For this review, take the finished solid that the model builds, in its own axes (mm). A direction names the side the tool comes from. Round coordinates to 2 decimals unless told otherwise and drop trailing zeros. Write each loop counter-clockwise with the first axis right and the second up, starting at its lowest first coordinate (ties: lowest second). Pieces come first, ordered by that corner, then holes. Notation, with made-up numbers: (28.5, 70.25) -> (74.5, 70.25) arc R4 ccw to (74.5, 76.25) -> close; hole circle Ø5 at (-18, 45.5). An arc over 180 degrees is marked (long way). Answer in a Markdown table with one row per item.
from build123d import *

# Parameters (mm, degrees)
CUT_EXTRUDE1_REACH      = 219.495
CUT_EXTRUDE1_END_RADIUS = 7.5
SKETCH2_W               = 8
SKETCH2_H               = 13
CUT_EXTRUDE2_REACH      = 219.495
CUT_EXTRUDE2_END_RADIUS = 7.5
SKETCH2_3_W             = 4.6
SKETCH2_3_H             = 13


with BuildPart() as part:
    # Sketch1 → Revolve1 (revolve)
    with BuildSketch(Plane.XY, mode=Mode.PRIVATE) as revolve1_sk:
        Polygon((157, 6.5), (157, 7.5), (55, 7.5), (55, 18), (-55, 18), (-55, 7.5), (-216, 7.5), (-216, 6.5), align=None)
    revolve(revolve1_sk.sketch.rotate(Axis((196.356223274, 0, 0), (-1, 0, 0)), 90), axis=Axis((196.356223274, 0, 0), (-1, 0, 0)))

    # Cut-Extrude1: up to this cylinder (the profile starts inside it)
    cut_extrude1_end = Plane(origin=(-64, 0, 0), z_dir=(1, 0, 0)) * Cylinder(CUT_EXTRUDE1_END_RADIUS, 454.99, mode=Mode.PRIVATE)
    # Sketch2 → Cut-Extrude1 (cut, up to the surface)
    with BuildSketch(Plane(origin=(0, 0, 0), x_dir=(1, 0, 0), z_dir=(0, 1, 0)), mode=Mode.PRIVATE) as cut_extrude1_sk1:
        with Locations((-64, 0)):
            Rectangle(SKETCH2_W, SKETCH2_H)
    cut_extrude1_tool1 = extrude(cut_extrude1_sk1.sketch, amount=-CUT_EXTRUDE1_REACH, mode=Mode.PRIVATE) & cut_extrude1_end
    add(cut_extrude1_tool1.solids().sort_by_distance((-64, 0, 0))[0], mode=Mode.SUBTRACT)

    # Cut-Extrude2: up to this cylinder (the profile starts inside it)
    cut_extrude2_end = Plane(origin=(-183.3, 0, 0), z_dir=(1, 0, 0)) * Cylinder(CUT_EXTRUDE2_END_RADIUS, 454.99, mode=Mode.PRIVATE)
    # Sketch2<3> → Cut-Extrude2 (cut, up to the surface)
    with BuildSketch(Plane(origin=(0, 0, 0), x_dir=(1, 0, 0), z_dir=(0, 1, 0)), mode=Mode.PRIVATE) as cut_extrude2_sk1:
        with Locations((-183.3, 0)):
            Rectangle(SKETCH2_3_W, SKETCH2_3_H)
    cut_extrude2_tool1 = extrude(cut_extrude2_sk1.sketch, amount=CUT_EXTRUDE2_REACH, mode=Mode.PRIVATE) & cut_extrude2_end
    add(cut_extrude2_tool1.solids().sort_by_distance((-183.3, 0, 0))[0], mode=Mode.SUBTRACT)


solid = part.part
1) Consider section A-A on z = 0. State the section outline as (x, y) points, then the cut area to 3 significant figures.
Solved:
| item | result |
|---|---|
| outline | (-216, -7.5) -> (-68, -7.5) -> (-68, -6.5) -> (-216, -6.5) -> close; (-216, 6.5) -> (-185.6, 6.5) -> (-185.6, 7.5) -> (-216, 7.5) -> close; (-181, 6.5) -> (157, 6.5) -> (157, 7.5) -> (55, 7.5) -> (55, 18) -> (-55, 18) -> (-55, 7.5) -> (-181, 7.5) -> close; (-60, -7.5) -> (-55, -7.5) -> (-55, -18) -> (55, -18) -> (55, -7.5) -> (157, -7.5) -> (157, -6.5) -> (-60, -6.5) -> close |
| area | 3,040 mm² |
2) Clearance check with flat-ended pins moving along their axes: pin 1 Ø6 at (x, z) = (34.5, -10) entering from -Y; pin 2 Ø4 at (x, y) = (-63, -2.5) entering from -Z; pin 3 Ø3 at (x, y) = (0, -12) entering from +Z; pin 4 Ø4 at (y, z) = (-2, -1.5) entering from -X. State where each tip first meets the part, or that it passes through.
Solved:
| item | result |
|---|---|
| pin 1 | y = -16.58 |
| pin 2 | z = -7.48 |
| pin 3 | z = 14.62 |
| pin 4 | through |
3) For line 1 (Y direction, x = 76, z = 0); line 2 (X direction, y = 4, z = 6); line 3 (Y direction, x = 33, z = 0), list the stretches that pass through material, from the lowest coordinate up. Write a range as [from, to].
Solved:
| item | result |
|---|---|
| line 1 | [-7.5, -6.5], [6.5, 7.5] |
| line 2 | [-216, -185.6], [-181, 157] |
| line 3 | [-18, -6.5], [6.5, 18] |
4) For faces 1 (the flat face through (-60, -7, 0)), 2 (the cylindrical face through (105.286, -6.324, -4.032)), 3 (the flat face through (-55, 8, 0)), 4 (the flat face through (-185.6, 7, 0)), list the 3-axis set-ups (+Z, -Z, +X, -X, +Y, -Y) from which the entire face can be reached by the end or side of a thin tool; tool diameter is ignored.
Solved:
| item | result |
|---|---|
| face 1 | -Y |
| face 2 | +X |
| face 3 | -X |
| face 4 | +Y |
5) Mouldability with a two-part tool opening along Z and no side actions: class faces 5 (the flat face through (157, -3, -6)), 6 (the flat face through (-68, -7, 0)), 7 (the cylindrical face through (-136.63, 7.32, 1.63)) as pulls with the +Z half, pulls with the -Z half, needs draft (parallel to the pull), parting line crosses it, or undercut.
Solved:
| item | result |
|---|---|
| face 5 | needs draft |
| face 6 | undercut |
| face 7 | parting line crosses it |
6) Consider section B-B on x = -35. State the section outline as (y, z) points.
Solved:
| item | result |
|---|---|
| outline | circle Ø36 at (0, 0); hole circle Ø13 at (0, 0) |
7) Consider section C-C on x = -111. State the section outline as (y, z) points, then the cut area to 3 significant figures.
Solved:
| item | result |
|---|---|
| outline | circle Ø15 at (0, 0); hole circle Ø13 at (0, 0) |
| area | 44.0 mm² |
